Source: CAD feature listing. Evaluate the final solid. Frame: model axes, mm. A direction names the side the tool comes from. Give positions to 0.01 mm unless a question says otherwise; leave off trailing zeros. Write each loop counter-clockwise with the first axis right and the second up, starting at its lowest first coordinate (ties: lowest second). Pieces come first, ordered by that corner, then holes. Notation, with made-up numbers: (22.5, 18) - (43.5, 18) arc R17 cw to (43.5, 34) - close; hole circle Ø8 at (70, 75). An arc over 180 degrees is marked (long way). Answer as a JSON object with one key per item and string values. Group by question number.
from build123d import *

# Parameters (mm, degrees)
F0_R          = 3.625
F0_R_2        = 2.375
F1_DEPTH      = 1
F1_DEPTH_BACK = 2
F2_DEPTH      = 7
F4_DEPTH      = 0.75


with BuildPart() as f1:
    # F0 (on Front) → F1 (new body, two sides)
    with BuildSketch(Plane.XZ) as f1_sk:
        Circle(F0_R)
        Circle(F0_R_2, mode=Mode.SUBTRACT)
    extrude(amount=F1_DEPTH)
    extrude(f1_sk.sketch, amount=-F1_DEPTH_BACK)

    # F0 (on Front) → F2 (join)
    with BuildSketch(Plane.XZ):
        Circle(F0_R_2)
    extrude(amount=F2_DEPTH)

    # F3 (on Right) → F4 (join, symmetric)
    with BuildSketch(Plane.YZ):
        Polygon((1.5, 3.5), (2, 3.5), (2, 7), (1.5, 7), (1.5, 6), align=None)
        Polygon((0.5, 6), (1.5, 6), (1.5, 7), align=None)
    extrude(amount=F4_DEPTH, both=True)


solid = f1.part
Q1. Ray query, probe 1 along Z at (x, y) = (0, 0.75) (3 decimals); probe 2 along Z at (x, y) = (0, 1.1) (3 decimals); probe 3 along X at (y, z) = (0.25, 0.25). Return the intervals inside material, ascending. Write a range as [from, to].
Q2. Section D-D on y = -0.5. Return the cut outline in (x, z) (3 decimals).
Q3. Section A-A on y = 0.75. Return the cut outline in (x, z) (3 decimals).
Q4. First-contact query: pin 1 Ø0.5 at (y, z) = (1.5, 5) entering from +X; pin 2 Ø5 at (y, z) = (-5.5, 0) entering from -X (3 decimals); pin 3 Ø1.2 at (y, z) = (1.5, 5.5) entering from -X. Flat tips, straight axial feed; report the tip coordinate or a pass-through.
Q5. Draft query along Z for faces 5 (the flat face through (0.8, -1, -2.4)), 6 (the flat face through (0, 1, 6.5)), 7 (the cylindrical face through (1.096, -3.958, -2.107)), 8 (the flat face through (0, 0, 0)). Return one class per face: released by +Z, released by -Z, zero draft, split by the parting line, or undercut.
Q6. Reachability of faces 1 (the cylindrical face through (1.096, 0.986, -2.107)), 2 (the flat face through (0, 1, 6)), 3 (the flat face through (0.75, 1.7, 5.7)), 4 (the flat face through (-0.75, 1.7, 5.7)) from +Z, -Z, +X, -X, +Y, -Y: full face, straight path, thin tool, end or side. Return the list, or none.
Q7. Section C-C on x = 0. Return the cut outline in (y, z) (3 decimals).
Q8. Section B-B on z = 0. Return the cut outline in (x, y) (3 decimals), then the cut area to 4 significant figures.
Taken from the geometry:
{
 "1": {"probe 1": "z = [-3.625, -2.375], [2.375, 3.625], [6, 6.25]", "probe 2": "z = [-3.625, -2.375], [2.375, 3.625], [6, 6.6]", "probe 3": "x = [-3.62, -2.36], [2.36, 3.62]"},
 "2": {"outline": "circle Ø7.25 at (0, 0)"},
 "3": {"outline": "circle Ø7.25 at (0, 0); (-0.75, 6) - (0.75, 6) - (0.75, 6.25) - (-0.75, 6.25) - close; hole circle Ø4.75 at (0, 0)"},
 "4": {"pin 1": "stops at x = 0.75", "pin 2": "stops at x = -2.375", "pin 3": "stops at x = -0.75"},
 "5": {"face 5": "zero draft", "face 6": "released by +Z", "face 7": "split by the parting line", "face 8": "undercut"},
 "6": {"face 1": "+Y", "face 2": "+X, -X, -Y", "face 3": "+Z, +X, +Y, -Y", "face 4": "+Z, -X, +Y, -Y"},
 "7": {"outline": "(-7, -2.375) - (-1, -2.375) - (-1, -3.625) - (2, -3.625) - (2, -2.375) - (0, -2.375) - (0, 2.375) - (2, 2.375) - (2, 7) - (1.5, 7) - (0.5, 6) - (1.5, 6) - (1.5, 3.625) - (-1, 3.625) - (-1, 2.375) - (-7, 2.375) - close"},
 "8": {"outline": "(-3.625, -1) - (-2.375, -1) - (-2.375, -7) - (2.375, -7) - (2.375, -1) - (3.625, -1) - (3.625, 2) - (2.375, 2) - (2.375, 0) - (-2.375, 0) - (-2.375, 2) - (-3.625, 2) - close", "area": "40.75 mm²"}
}
